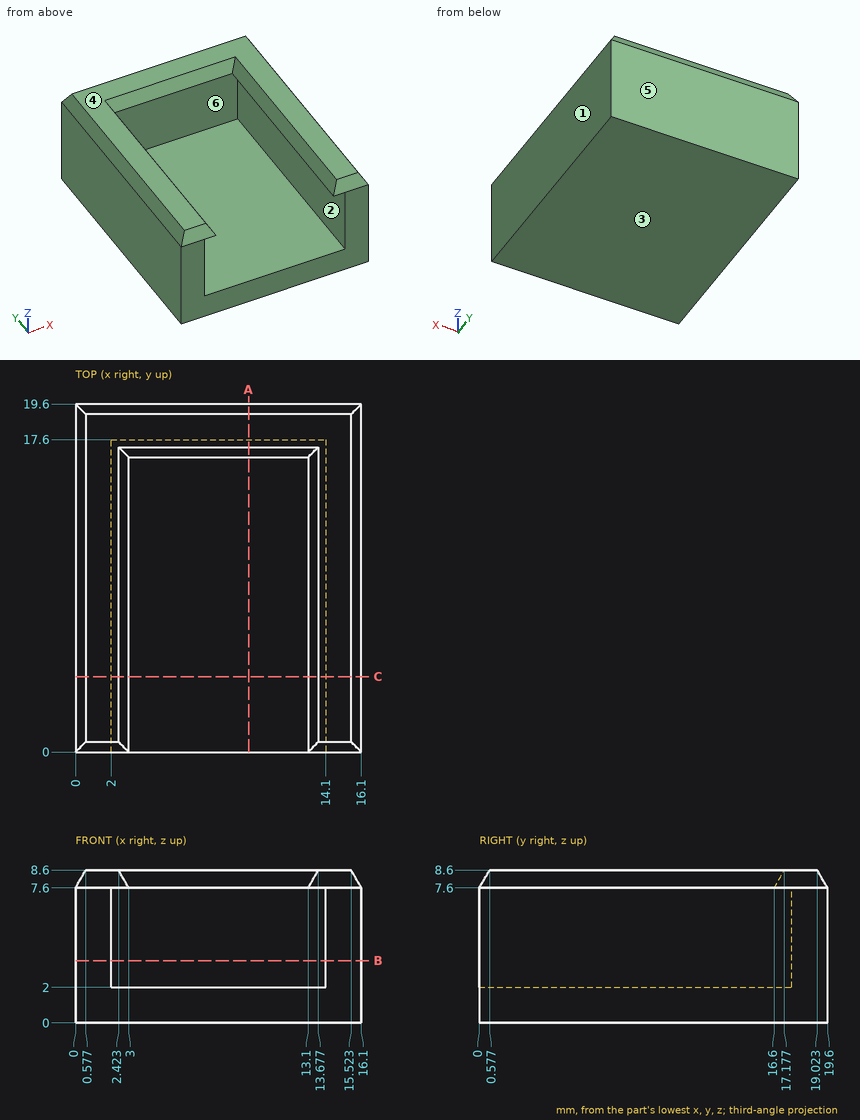
Source: three-view drawing plus pictorial views. Frame: mm from the lowest corner of the part. A direction names the side the tool comes from. Round coordinates to 2 decimals unless told otherwise and drop trailing zeros. Loops run counter-clockwise (first coordinate to the right, second up) from the corner with the lowest first, then second, coordinate; pieces in that order, holes last.
1. Mould query, pull axis Z, two halves, no side actions, for the marked faces 3, 4, 5 and 6. Classes: released by +Z, released by -Z, zero draft, split by the parting line, or undercut.
2. Section query B-B on z = 3.5. Output: boundary loops of the cut face in (x, y), and give its area (3 significant figures).
3. Ray query, L1, parallel to Z at x = 13.75, y = 1.5; L2, parallel to X at y = 5.25, z = 3; L3, parallel to Y at x = 7.5, z = 5.75. Return the intervals inside material, ascending.
4. Section query C-C on y = 4.25. Output: boundary loops of the cut face in (x, z).
5. Section query A-A on x = 9.75. Output: boundary loops of the cut face in (y, z).
6. Access query for the marked faces 1 and 2. Directions: +Z, -Z, +X, -X, +Y, -Y. A direction counts if a zero-diameter tool reaches every point of the face in a straight line with its end or side. Return the directions, or none.
7. Contact query for flat-ended pins moving along their axis: pin 1 (1.7 mm diameter, centred on x = 5.5, z = 5.5, fed in from -Y); pin 2 (1.5 mm diameter, centred on x = 5, y = 5, fed in from +Z). Output: stop coordinate, or through.
Answers below:
1. face 3: released by -Z
1. face 4: released by +Z
1. face 5: zero draft
1. face 6: undercut
2. outline: (0, 0) - (2, 0) - (2, 17.6) - (14.1, 17.6) - (14.1, 0) - (16.1, 0) - (16.1, 19.6) - (0, 19.6) - close
2. area: 103 mm2
3. L1: z = 0 to 2, 7.6 to 8.6
3. L2: x = 0 to 2, 14.1 to 16.1
3. L3: y = 17.6 to 19.6
4. outline: (0, 0) - (16.1, 0) - (16.1, 7.6) - (15.52, 8.6) - (13.68, 8.6) - (13.1, 7.6) - (14.1, 7.6) - (14.1, 2) - (2, 2) - (2, 7.6) - (3, 7.6) - (2.42, 8.6) - (0.58, 8.6) - (0, 7.6) - close
5. outline: (0, 0) - (19.6, 0) - (19.6, 7.6) - (19.02, 8.6) - (17.18, 8.6) - (16.6, 7.6) - (17.6, 7.6) - (17.6, 2) - (0, 2) - close
6. face 1: +Z, -Z, +X, +Y, -Y
6. face 2: -Y
7. pin 1: stops at y = 17.6
7. pin 2: stops at z = 2
